The model under review builds one solid part; all positions refer to its coordinate system, in mm. A direction names the side the tool comes from. Round coordinates to 2 decimals unless told otherwise and drop trailing zeros. Loops run counter-clockwise (first coordinate to the right, second up) from the corner with the lowest first, then second, coordinate; pieces in that order, holes last. Notation, with made-up numbers: M -5.75,41.5 L 48.25,41.5 A30 ccw 48.25,74.5 Z; hole C -36,65 d1. An arc over 180 degrees is marked long. Return JSON: item names as keys, results as strings. Group by question number.
Q1. Consider section C-C (x = -28.5). State the section outline as (y, z) points.
Q2. Draft analysis for pull direction Y (two halves, no side actions). For faces 4 (the face through (40.924, -22.066, 2.028)), 5 (the face through (-53.34, 8.97, 1.97)), 6 (the face through (58, 57, -12)), 7 (the face through (92.48, 55.03, -7.33)), state which applies: pulls with the +Y half, pulls with the -Y half, needs draft (parallel to the pull), parting line crosses it, or undercut.
Q3. Consider section B-B (x = 102). State the section outline as (y, z) points, and give its area (3 significant figures).
Q4. Consider section A-A (z = -7). State the section outline as (x, y) points.
Q5. For faces 1 (the face through (60, -40, 2)), 2 (the face through (58, 53, -12)), 3 (the face through (173.34, 8.97, 1.97)), list the 3-axis set-ups (+Z, -Z, +X, -X, +Y, -Y) from which the entire face can be reached by the end or side of a thin tool; tool diameter is ignored.
Q6. To check wall thickness, follow line 1 along X through (y, z) = (55.75, -16); line 2 along X through (y, z) = (-45, 3.15); line 3 along Y through (x, z) = (147, -13.25). State the ranges of each line that lie inside material, in increasing order.
Q7. Clearance check with flat-ended pins moving along their axes: pin 1 Ø3 at (x, y) = (0, -45) entering from +Z (3 decimals); pin 2 Ø3 at (x, y) = (67.5, -32.5) entering from -Z; pin 3 Ø6 at (x, z) = (149, -9) entering from -Y; pin 4 Ø5 at (x, y) = (38.97, -22.5) entering from +Z. State where each tip first meets the part, or that it passes through.
from build123d import *

# Parameters (mm, degrees)
BOSS_EXTRUDE1_DEPTH                                 = 4
BOSS_EXTRUDE7_DEPTH                                 = 240
CIRPATTERN1_COUNT                                   = 5
CIRPATTERN1_ANGLE                                   = 240
BOSS_EXTRUDE5_DEPTH                                 = 4
FILLET4_R                                           = 5
CSK_FOR_M2_COUNTERSUNK_FLAT_HEAD_SCREW1_D           = 2.4
CSK_FOR_M2_COUNTERSUNK_FLAT_HEAD_SCREW1_DEPTH       = 9
CSK_FOR_M2_COUNTERSUNK_FLAT_HEAD_SCREW1_CSINK_D     = 4.4
CSK_FOR_M2_COUNTERSUNK_FLAT_HEAD_SCREW1_CSINK_ANGLE = 90
CSK_FOR_M2_COUNTERSUNK_FLAT_HEAD_SCREW1_TIP         = 0.721032743
CUT_EXTRUDE1_DEPTH                                  = 4
CUT_EXTRUDE2_DEPTH                                  = 240
F_5_0MM_DOWEL_HOLE2_AT_2_COUNT                      = 2
F_5_0MM_DOWEL_HOLE2_AT_2_PITCH                      = 9
LPATTERN2_COUNT                                     = 2
LPATTERN2_PITCH                                     = 65
FILLET7_R                                           = 10
BOSS_EXTRUDE8_DEPTH                                 = 4


with BuildPart() as part:
    # Sketch1 → Boss-Extrude1 (new body)
    with BuildSketch(Plane.XY):
        with BuildLine():
            Line((-65, 55), (65, 55))
            Line((65, 55), (46.854237316, -14.341563567))
            ThreePointArc((46.854237316, -14.341563567), (-0.646903027, -48.995729574), (-47.216548934, -13.099523151))
            Line((-47.216548934, -13.099523151), (-65, 51))
            Line((-65, 51), (-65, 55))
        make_face()
    boss_extrude1 = extrude(amount=BOSS_EXTRUDE1_DEPTH)

    # Sketch17 → Boss-Extrude7 (add)
    with BuildSketch(Plane(origin=(-60, 0, 0), x_dir=(0, 0, -1), z_dir=(1, 0, 0))):
        with BuildLine():
            Line((20, 53), (20, 57))
            Line((20, 57), (4, 57))
            ThreePointArc((4, 57), (-1.656854249, 54.656854249), (-4, 49))
            Line((-4, 49), (-4, 32.977760415))
            Line((-4, 32.977760415), (0, 32.977760415))
            Line((0, 32.977760415), (0, 49))
            ThreePointArc((0, 49), (1.171572875, 51.828427125), (4, 53))
            Line((4, 53), (20, 53))
        make_face()
    extrude(amount=BOSS_EXTRUDE7_DEPTH)

    # Mirror1: Boss-Extrude1 across plane
    add(boss_extrude1.mirror(Plane(origin=(60, 0, 0), x_dir=(0, 0, 1), z_dir=(1, 0, 0))))

    # Sketch3 → 4.0mm Dowel Hole1 (revolve, cut)
    with BuildSketch(Plane(origin=(0, 45, 4), x_dir=(0, -1, 0), z_dir=(1, 0, 0))):
        Polygon((0, 0), (0, 51.201721238), (2, 50), (2, 0), align=None)
    f_4_0mm_dowel_hole1 = revolve(axis=Axis((0, 45, 10.35), (0, 0, -1)), mode=Mode.SUBTRACT)

    # CirPattern1: 4.0mm Dowel Hole1 ×5 about axis
    cirpattern1_axis = Axis((0, 0, 0), (0, 0, -1))
    for i in range(1, CIRPATTERN1_COUNT):
        add(f_4_0mm_dowel_hole1.rotate(cirpattern1_axis, i * CIRPATTERN1_ANGLE / (CIRPATTERN1_COUNT - 1)), mode=Mode.SUBTRACT)

    # Mirror2: 4.0mm Dowel Hole1 across plane
    add(f_4_0mm_dowel_hole1.mirror(Plane(origin=(60, 0, 0), x_dir=(0, 0, 1), z_dir=(1, 0, 0))), mode=Mode.SUBTRACT)

    # Mirror2 copy 1 sketch → Mirror2 copy 1 (revolve, cut)
    with BuildSketch(Plane(origin=(81.02885683, 22.5, 4), x_dir=(0.8660254037844399, -0.4999999999999978, 0), z_dir=(-0.4999999999999978, -0.8660254037844399, 0))):
        Polygon((0, 0), (0, -51.201721238), (2, -50), (2, 0), align=None)
    revolve(axis=Axis((81.02885683, 22.5, 10.35), (0, 0, 1)), mode=Mode.SUBTRACT)

    # Mirror2 copy 2 sketch → Mirror2 copy 2 (revolve, cut)
    with BuildSketch(Plane(origin=(81.02885683, -22.5, 4), x_dir=(0.866025403784436, 0.5000000000000044, 0), z_dir=(0.5000000000000044, -0.866025403784436, 0))):
        Polygon((0, 0), (0, -51.201721238), (2, -50), (2, 0), align=None)
    revolve(axis=Axis((81.02885683, -22.5, 10.35), (0, 0, 1)), mode=Mode.SUBTRACT)

    # Mirror2 copy 3 sketch → Mirror2 copy 3 (revolve, cut)
    with BuildSketch(Plane(origin=(120, -45, 4), x_dir=(0, 1, 0), z_dir=(1, 0, 0))):
        Polygon((0, 0), (0, -51.201721238), (2, -50), (2, 0), align=None)
    revolve(axis=Axis((120, -45, 10.35), (0, 0, 1)), mode=Mode.SUBTRACT)

    # Mirror2 copy 4 sketch → Mirror2 copy 4 (revolve, cut)
    with BuildSketch(Plane(origin=(158.97114317, -22.5, 4), x_dir=(-0.8660254037844437, 0.4999999999999912, 0), z_dir=(0.4999999999999912, 0.8660254037844437, 0))):
        Polygon((0, 0), (0, -51.201721238), (2, -50), (2, 0), align=None)
    revolve(axis=Axis((158.97114317, -22.5, 10.35), (0, 0, 1)), mode=Mode.SUBTRACT)

    # Sketch11 → Boss-Extrude5 (add)
    with BuildSketch(Plane.XY.offset(4)):
        Polygon((28.301943396, -40), (91.698056604, -40), (77.749149407, -24.816640065), (71.110361187, 23.59948562), (49.712708472, 23.59948562), (42.81015603, -23.838845205), align=None)
    extrude(amount=-BOSS_EXTRUDE5_DEPTH)

    # Fillet4
    fillet4_edges = [part.edges().sort_by_distance(p)[0] for p in [
        (28.301943396, -40, 2),
        (91.698056604, -40, 2),
    ]]
    fillet(fillet4_edges, radius=FILLET4_R)

    # CSK for M2 Countersunk Flat Head Screw1
    with Locations(Plane.XY.offset(4)):
        with Locations((52.5, -32.5), (67.5, -32.5)):
            CounterSinkHole(CSK_FOR_M2_COUNTERSUNK_FLAT_HEAD_SCREW1_D / 2, CSK_FOR_M2_COUNTERSUNK_FLAT_HEAD_SCREW1_CSINK_D / 2, depth=CSK_FOR_M2_COUNTERSUNK_FLAT_HEAD_SCREW1_DEPTH, counter_sink_angle=CSK_FOR_M2_COUNTERSUNK_FLAT_HEAD_SCREW1_CSINK_ANGLE)
            with Locations((0, 0, -(CSK_FOR_M2_COUNTERSUNK_FLAT_HEAD_SCREW1_DEPTH + CSK_FOR_M2_COUNTERSUNK_FLAT_HEAD_SCREW1_TIP / 2))):  # 118° drill point
                Cone(0, CSK_FOR_M2_COUNTERSUNK_FLAT_HEAD_SCREW1_D / 2, CSK_FOR_M2_COUNTERSUNK_FLAT_HEAD_SCREW1_TIP, mode=Mode.SUBTRACT)

    # Sketch18 → Cut-Extrude1 (cut)
    with BuildSketch(Plane(origin=(0, 0, 0), x_dir=(-1, 0, 0), z_dir=(0, 0, -1))):
        Polygon((60, 55), (60, 32.977760415), (65, 51), (65, 55), align=None)
    cut_extrude1 = extrude(amount=-CUT_EXTRUDE1_DEPTH, mode=Mode.SUBTRACT)

    # Mirror6: Cut-Extrude1 across plane
    add(cut_extrude1.mirror(Plane(origin=(60, 0, 0), x_dir=(0, 0, 1), z_dir=(1, 0, 0))), mode=Mode.SUBTRACT)

    # Sketch19 → Cut-Extrude2 (cut)
    with BuildSketch(Plane.ZY.offset(60)):
        with BuildLine():
            Line((1.291502622, 55), (4, 55))
            Line((4, 55), (4, 49))
            ThreePointArc((4, 49), (3.291502622, 52.291502622), (1.291502622, 55))
        make_face()
    extrude(amount=-CUT_EXTRUDE2_DEPTH, mode=Mode.SUBTRACT)

    # Sketch21 → 5.0mm Dowel Hole2 (revolve, cut)
    with BuildSketch(Plane(origin=(-35, 57, -7), x_dir=(0, 0, 1), z_dir=(1, 0, 0))):
        Polygon((0, 0), (0, 10.502151548), (2.5, 9), (2.5, 0), align=None)
    f_5_0mm_dowel_hole2 = revolve(axis=Axis((-35, 63.35, -7), (0, -1, 0)), mode=Mode.SUBTRACT)

    # 5.0mm Dowel Hole2 at 2: 5.0mm Dowel Hole2 ×2
    with Locations(*[(0, 0, -i * F_5_0MM_DOWEL_HOLE2_AT_2_PITCH) for i in range(1, F_5_0MM_DOWEL_HOLE2_AT_2_COUNT)]):
        add(f_5_0mm_dowel_hole2, mode=Mode.SUBTRACT)

    # LPattern2: 5.0mm Dowel Hole2 ×2
    with Locations(*[(i * LPATTERN2_PITCH, 0, 0) for i in range(1, LPATTERN2_COUNT)]):
        add(f_5_0mm_dowel_hole2, mode=Mode.SUBTRACT)

    # LPattern2 copy 1 sketch → LPattern2 copy 1 (revolve, cut)
    with BuildSketch(Plane(origin=(30, 57, -16), x_dir=(0, 0, 1), z_dir=(1, 0, 0))):
        Polygon((0, 0), (0, 10.502151548), (2.5, 9), (2.5, 0), align=None)
    revolve(axis=Axis((30, 63.35, -16), (0, -1, 0)), mode=Mode.SUBTRACT)

    # Mirror7: 5.0mm Dowel Hole2 across plane
    add(f_5_0mm_dowel_hole2.mirror(Plane(origin=(60, 0, 0), x_dir=(0, 0, 1), z_dir=(1, 0, 0))), mode=Mode.SUBTRACT)

    # Mirror7 copy 1 sketch → Mirror7 copy 1 (revolve, cut)
    with BuildSketch(Plane(origin=(155, 57, -16), x_dir=(0, 0, 1), z_dir=(-1, 0, 0))):
        Polygon((0, 0), (0, -10.502151548), (2.5, -9), (2.5, 0), align=None)
    revolve(axis=Axis((155, 63.35, -16), (0, 1, 0)), mode=Mode.SUBTRACT)

    # Mirror7 copy 2 sketch → Mirror7 copy 2 (revolve, cut)
    with BuildSketch(Plane(origin=(90, 57, -7), x_dir=(0, 0, 1), z_dir=(-1, 0, 0))):
        Polygon((0, 0), (0, -10.502151548), (2.5, -9), (2.5, 0), align=None)
    revolve(axis=Axis((90, 63.35, -7), (0, 1, 0)), mode=Mode.SUBTRACT)

    # Mirror7 copy 3 sketch → Mirror7 copy 3 (revolve, cut)
    with BuildSketch(Plane(origin=(90, 57, -16), x_dir=(0, 0, 1), z_dir=(-1, 0, 0))):
        Polygon((0, 0), (0, -10.502151548), (2.5, -9), (2.5, 0), align=None)
    revolve(axis=Axis((90, 63.35, -16), (0, 1, 0)), mode=Mode.SUBTRACT)

    # Fillet7
    fillet7_edges = [part.edges().sort_by_distance(p)[0] for p in [
        (-60, 32.977760415, 2),
        (180, 32.977760415, 2),
    ]]
    fillet(fillet7_edges, radius=FILLET7_R)

    # Sketch22 → Boss-Extrude8 (add)
    with BuildSketch(Plane(origin=(0, 0, 0), x_dir=(-1, 0, 0), z_dir=(0, 0, -1))):
        Polygon((-63.217095964, 23.59948562), (-56.782904036, 23.59948562), (-59.237073514, 32.977760415), (-60.762926486, 32.977760415), align=None)
    extrude(amount=-BOSS_EXTRUDE8_DEPTH)


solid = part.part
Values:
{
 "1": {"outline": "M -39.86,0 L 49,0 A4 cw 53,-4 L 53,-20 L 57,-20 L 57,-4 A8 ccw 49,4 L -39.86,4 Z"},
 "2": {"face 4": "undercut", "face 5": "pulls with the -Y half", "face 6": "pulls with the +Y half", "face 7": "needs draft"},
 "3": {"outline": "M -45.57,0 L 49,0 A4 cw 53,-4 L 53,-20 L 57,-20 L 57,-4 A8 ccw 49,4 L -45.57,4 Z", "area": "480 mm2"},
 "4": {"outline": "M -60,53 L -37.5,53 L -37.5,57 L -60,57 Z; M -32.5,53 L 27.5,53 L 27.5,57 L -32.5,57 Z; M 32.5,53 L 87.5,53 L 87.5,57 L 32.5,57 Z; M 92.5,53 L 152.5,53 L 152.5,57 L 92.5,57 Z; M 157.5,53 L 180,53 L 180,57 L 157.5,57 Z"},
 "5": {"face 1": "+Z, -Z, -Y", "face 2": "-Z, +X, -X, -Y", "face 3": "+Z, -Z, +X, -Y"},
 "6": {"line 1": "x = -60 to -37.5, -32.5 to 27.5, 32.5 to 87.5, 92.5 to 152.5, 157.5 to 180", "line 2": "x = -19.39 to -2, 2 to 19.39, 100.61 to 118, 122 to 139.39", "line 3": "y = 53 to 57"},
 "7": {"pin 1": "passes through", "pin 2": "stops at z = 0", "pin 3": "stops at y = 53", "pin 4": "stops at z = 4"}
}
